from build123d import *

# Parameters (mm, degrees)
SKETCH1_R           = 1.65
BOSS_EXTRUDE1_DEPTH = 6
SKETCH2_W           = 15
SKETCH2_H           = 25
SKETCH2_R           = 3.15
BOSS_EXTRUDE2_DEPTH = 20
CUT_EXTRUDE1_DEPTH  = 52.537692211
SKETCH5_R           = 5.5
CUT_EXTRUDE2_DEPTH  = 62.80841078


with BuildPart() as part:
    # Sketch1 → Boss-Extrude1 (new body)
    with BuildSketch(Plane(origin=(0, 0, 0), x_dir=(1, 0, 0), z_dir=(0, 1, 0))):
        Polygon((-17.5, -7.5), (17.5, -7.5), (17.5, 7.5), (17.50136804, 16.71166189), (-42.49863196, 16.71166189), (-42.49863196, 1.71166189), align=None)
        with Locations(Location((-13, 0, 0), (0, 0, 270))):
            Circle(SKETCH1_R, mode=Mode.SUBTRACT)
        with Locations(Location((13, 0, 0), (0, 0, 270))):
            Circle(SKETCH1_R, mode=Mode.SUBTRACT)
    extrude(amount=BOSS_EXTRUDE1_DEPTH)

    # Sketch2 → Boss-Extrude2 (add)
    with BuildSketch(Plane.ZY.offset(42.49863196)):
        with Locations((-9.21166189, 12.5)):
            Rectangle(SKETCH2_W, SKETCH2_H)
        with Locations((-9.21166189, 19)):
            Circle(SKETCH2_R, mode=Mode.SUBTRACT)
    extrude(amount=-BOSS_EXTRUDE2_DEPTH)

    # Sketch4 → Cut-Extrude1 (cut, through all)
    with BuildSketch(Plane.XY.offset(-1.71166189)):
        Polygon((-36.49863196, 25), (-22.49863196, 6), (-22.49863196, 25), align=None)
    extrude(amount=-CUT_EXTRUDE1_DEPTH, mode=Mode.SUBTRACT)

    # Sketch5 → Cut-Extrude2 (cut, through all)
    with BuildSketch(Plane.ZY.offset(36.49863196)):
        with Locations((-9.21166189, 19)):
            Circle(SKETCH5_R)
    extrude(amount=-CUT_EXTRUDE2_DEPTH, mode=Mode.SUBTRACT)


solid = part.part
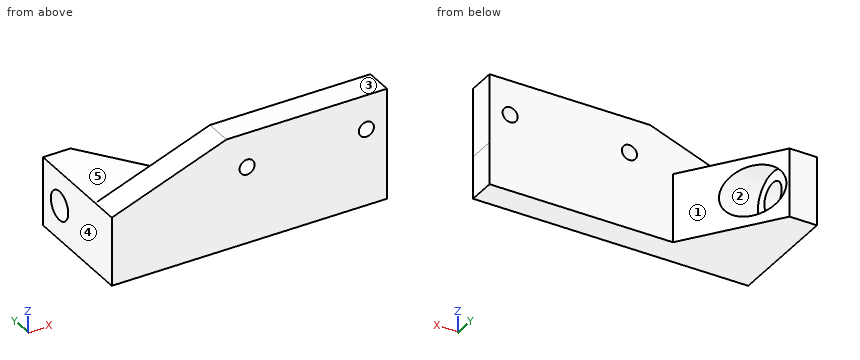
Source: CAD feature listing. Evaluate the final solid. Frame: model axes, mm. Face numbers are marked on the shaded views. A direction names the side the tool comes from. Coordinates: 2 decimals unless noted, no trailing zeros. Order: outer loops, then holes, each group sorted by start corner. A loop starts at its lowest first (then second) coordinate and runs counter-clockwise, first axis right, second up. Notation, with made-up numbers: M 74,14 L 113,14 A23 cw 113,50 Z; hole C 45.25,-19 d7. An arc over 180 degrees is marked long. Write each question's results on one line, items separated by ' | '. Start each with the question number.
1. Section B-B, the plane y = 19. Return the cut outline in (x, z), then the cut area to 3 significant figures.
2. Material intervals for L1, parallel to Z at x = -29.5, y = 14.5; L2, parallel to Y at x = -8.5, z = -10.5; L3, parallel to Z at x = -32.75, y = 19, sorted ascending.
3. Section D-D, the plane z = -13.5. Return the cut outline in (x, y).
4. Section C-C, the plane x = -16. Return the cut outline in (y, z), then the cut area to 3 significant figures.
5. Draft query along Z for the marked faces 1, 2 and 3. Return one class per face: +Z half, -Z half, draft (parallel to the pull), parting line (faces both ways), or undercut.
6. Reachability of the marked faces 4 and 5 from +Z, -Z, +X, -X, +Y, -Y: full face, straight path, thin tool, end or side. Return the list, or none.
7. Pin query (flat end, axial travel): pin 1 (8 mm diameter, centred on x = -22.5, z = 4.5, fed in from +Y); pin 2 (9 mm diameter, centred on y = 17, z = -11, fed in from +X); pin 3 (4 mm diameter, centred on x = -23, z = -7.5, fed in from +Y). Return the tip coordinate at first contact, or that it passes through.
8. Section A-A, the plane x = 13. Return the cut outline in (y, z).
Solution:
1) outline: M -42.5,-16.71 L -32.08,-16.71 L -32.08,-14.71 L -36.5,-14.71 L -36.5,-12.36 L -42.5,-12.36 Z; M -42.5,-6.06 L -36.5,-6.06 L -36.5,-3.71 L -32.08,-3.71 L -32.08,-1.71 L -42.5,-1.71 Z | area: 69.9 mm²
2) L1: -16.71 to -12.37, -6.05 to -1.71 | L2: 0 to 6 | L3: -16.71 to -14.71, -3.71 to -1.71
3) outline: M -42.5,0 L 17.5,0 L 17.5,6 L -22.5,6 L -29.54,15.56 L -36.5,15.56 L -36.5,22.44 L -34.62,22.44 L -36.5,25 L -42.5,25 Z
4) outline: M 0,-16.71 L 6,-16.71 L 6,7.5 L 0,7.5 Z | area: 145 mm²
5) face 1: draft | face 2: undercut | face 3: +Z half
6) face 4: +Z, -Z, -X, +Y, -Y | face 5: +Z, +X, -X, +Y
7) pin 1: y = 6 | pin 2: x = -27.29 | pin 3: y = 9.39
8) outline: M 0,-16.71 L 6,-16.71 L 6,-1.65 L 0,-1.65 Z; M 0,1.65 L 6,1.65 L 6,7.5 L 0,7.5 Z
